Geometry check sheet. Reference: the model listing, model coordinates, mm. Face numbers are marked on the shaded views. A direction names the side the tool comes from. Coordinates: 2 decimals unless noted, no trailing zeros. Write each loop counter-clockwise with the first axis right and the second up, starting at its lowest first coordinate (ties: lowest second). Pieces come first, ordered by that corner, then holes. Notation, with made-up numbers: (19.5, 10.25) -> (38.5, 10.25) arc R24 cw to (38.5, 23.25) -> close; hole circle Ø6 at (77, -21). An arc over 180 degrees is marked (long way). Answer in a Markdown table with one row per item. Add a question column.
Q1. Section check B-B, the plane y = 0. Record the boundary of the cut face in (x, z).
Q2. Section check A-A, the plane x = 0. Record the boundary of the cut face in (y, z).
Q3. Release check for a two-part mould opening along X. For the marked faces 3 and 4 record: pulls with the +X half, pulls with the -X half, needs draft (parallel to the pull), parting line crosses it, or undercut.
Q4. Tool access check on the marked faces 1 and 2. Record the directions out of +Z, -Z, +X, -X, +Y, -Y that give a thin tool (end or side, any length) a straight path to the whole face; none if there is none.
Q5. Section check C-C, the plane z = 24. Record the boundary of the cut face in (x, y).
Q6. Gauge pin test, flat ends, axial feed: P1, Ø1, axis at x = -2.5, z = 10, coming from the -Y side; P2, Ø1.5, axis at x = 2, y = -8.5, coming from the +Z side; P3, Ø12, axis at y = -5, z = 19.5, coming from the -X side. Record the tip position at first contact, or that the pin passes through.
Q7. Thickness scan on line 1 (Z direction, x = -6, y = -4.5); line 2 (Y direction, x = 0.5, z = 22.5); line 3 (Y direction, x = 3.25, z = 5.5). Record the ranges inside material, lowest first.
Q8. Section check D-D, the plane x = 4. Record the boundary of the cut face in (y, z).
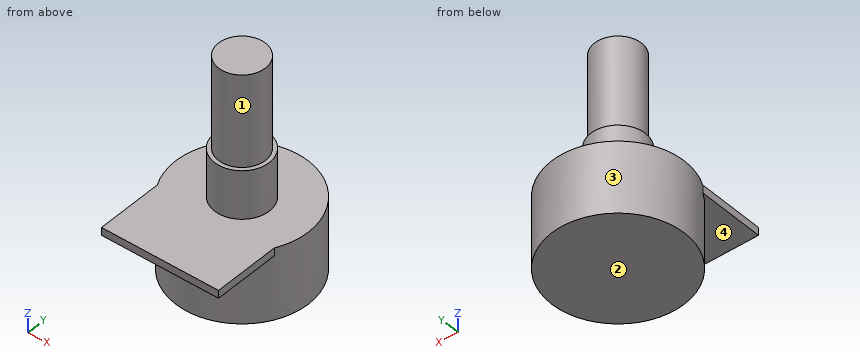
```python
from build123d import *

# Parameters (mm, degrees)
SCHIZZO1_R                   = 8.5
ESTRUSIONE_ESTRUSIONE1_DEPTH = 9.2
SCHIZZO2_W                   = 15
SCHIZZO2_H                   = 8.5
ESTRUSIONE_ESTRUSIONE2_DEPTH = 1
SCHIZZO3_R                   = 3.5
ESTRUSIONE_ESTRUSIONE3_DEPTH = 6.2
SCHIZZO4_R                   = 3
ESTRUSIONE_ESTRUSIONE4_DEPTH = 11.8


with BuildPart() as part:
    # Schizzo1 → Estrusione-Estrusione1 (new body)
    with BuildSketch(Plane.XY):
        Circle(SCHIZZO1_R)
    extrude(amount=ESTRUSIONE_ESTRUSIONE1_DEPTH)

    # Schizzo2 → Estrusione-Estrusione2 (add)
    with BuildSketch(Plane.XY.offset(9.2)):
        with Locations((0, -8.25)):
            Rectangle(SCHIZZO2_W, SCHIZZO2_H)
    extrude(amount=-ESTRUSIONE_ESTRUSIONE2_DEPTH)

    # Schizzo3 → Estrusione-Estrusione3 (add)
    with BuildSketch(Plane.XY.offset(9.2)):
        with Locations(Location((0, 0, 0), (0, 0, 180))):
            Circle(SCHIZZO3_R)
    extrude(amount=ESTRUSIONE_ESTRUSIONE3_DEPTH)

    # Schizzo4 → Estrusione-Estrusione4 (add)
    with BuildSketch(Plane.XY.offset(15.4)):
        Circle(SCHIZZO4_R)
    extrude(amount=ESTRUSIONE_ESTRUSIONE4_DEPTH)


solid = part.part
```
Calculated:
| question | item | result |
|---|---|---|
| 1 | outline | (-8.5, 0) -> (8.5, 0) -> (8.5, 9.2) -> (3.5, 9.2) -> (3.5, 15.4) -> (3, 15.4) -> (3, 27.2) -> (-3, 27.2) -> (-3, 15.4) -> (-3.5, 15.4) -> (-3.5, 9.2) -> (-8.5, 9.2) -> close |
| 2 | outline | (-12.5, 8.2) -> (-8.5, 8.2) -> (-8.5, 0) -> (8.5, 0) -> (8.5, 9.2) -> (3.5, 9.2) -> (3.5, 15.4) -> (3, 15.4) -> (3, 27.2) -> (-3, 27.2) -> (-3, 15.4) -> (-3.5, 15.4) -> (-3.5, 9.2) -> (-12.5, 9.2) -> close |
| 3 | face 3 | parting line crosses it |
| 3 | face 4 | needs draft |
| 4 | face 1 | +Z |
| 4 | face 2 | -Z, +X, -X, +Y, -Y |
| 5 | outline | circle Ø6 at (0, 0) |
| 6 | P1 | stops at y = -2.87 |
| 6 | P2 | stops at z = 9.2 |
| 6 | P3 | stops at x = -3.44 |
| 7 | line 1 | z = 0 to 9.2 |
| 7 | line 2 | y = -2.96 to 2.96 |
| 7 | line 3 | y = -7.85 to 7.85 |
| 8 | outline | (-12.5, 8.2) -> (-7.5, 8.2) -> (-7.5, 0) -> (7.5, 0) -> (7.5, 9.2) -> (-12.5, 9.2) -> close |
